Geometry check sheet. Reference: drawing and pictorial views, mm from the part's lowest x, y, z. Give positions to 0.01 mm unless a question says otherwise; leave off trailing zeros. Write each loop counter-clockwise with the first axis right and the second up, starting at its lowest first coordinate (ties: lowest second). Pieces come first, ordered by that corner, then holes. Notation, with made-up numbers: (-9.75, -20) -> (1.25, -20) arc R13 cw to (1.25, 0) -> close; hole circle Ø5 at (37.25, -23.5). An arc over 180 degrees is marked (long way). Write each question's results on one line, items separated by ' | '. Start each with the question number.
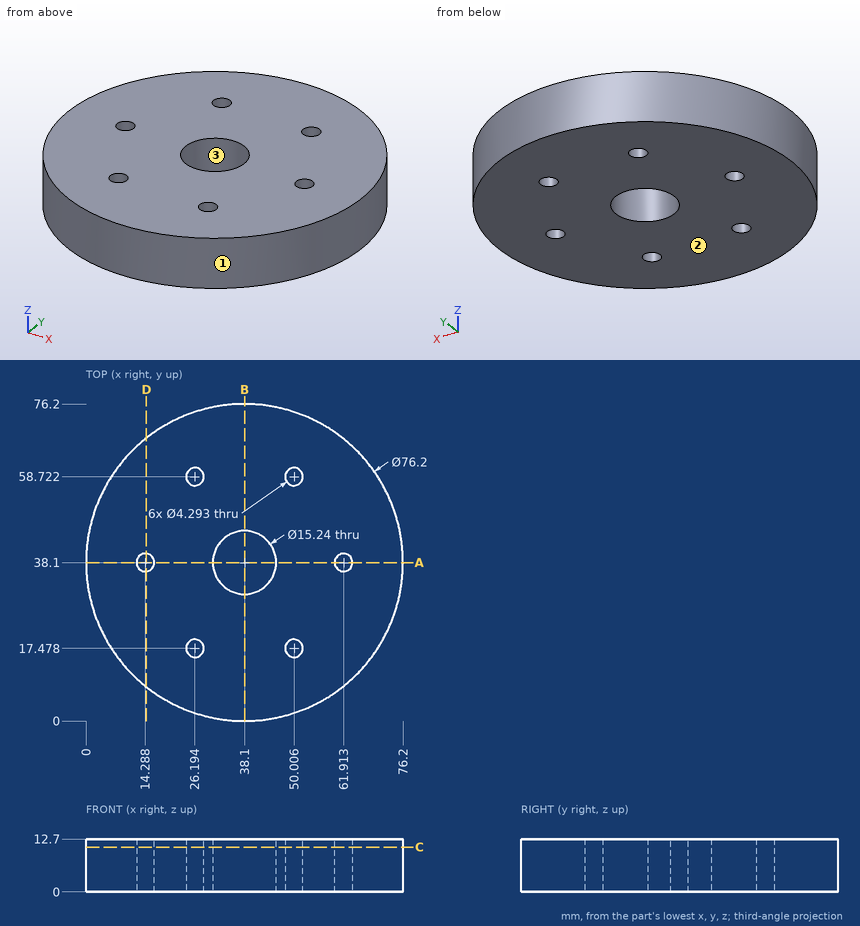
Item 1: Section check B-B on x = 38.1. Record the boundary of the cut face in (y, z).
Item 2: Section check D-D on x = 14.5. Record the boundary of the cut face in (y, z) (1 decimal).
Item 3: Depth check by flat-ended pin: pin 1 Ø4 at (x, z) = (27, 2) entering from -Y; pin 2 Ø3.5 at (x, y) = (50.01, 58.72) entering from -Z; pin 3 Ø5 at (x, y) = (50.01, 17.48) entering from -Z; pin 4 Ø1 at (y, z) = (52, 1.5) entering from -X (1 decimal). Enter the tip coordinate at first touch or a pass-through.
Item 4: Mould release check, pull along X, two halves, no side actions. Record for the marked faces 1, 2 and 3: pulls with the +X half, pulls with the -X half, needs draft (parallel to the pull), parting line crosses it, or undercut.
Item 5: Section check C-C on z = 10.75. Record the boundary of the cut face in (x, y).
Item 6: Section check A-A on y = 38.1. Record the boundary of the cut face in (x, z).
Item 7: Thickness scan on probe 1 along Y at (x, z) = (38, 4.5); probe 2 along X at (y, z) = (19, 11.75) (1 decimal); probe 3 along Y at (x, z) = (27, 8.5). Record the ranges inside material, lowest first. Write a range as from..to.
Check sheet entries:
1) outline: (0, 0) -> (30.48, 0) -> (30.48, 12.7) -> (0, 12.7) -> close; (45.72, 0) -> (76.2, 0) -> (76.2, 12.7) -> (45.72, 12.7) -> close
2) outline: (8.2, 0) -> (36, 0) -> (36, 12.7) -> (8.2, 12.7) -> close; (40.2, 0) -> (68, 0) -> (68, 12.7) -> (40.2, 12.7) -> close
3) pin 1: stops at y = 1.1 | pin 2: passes through | pin 3: stops at z = 0 | pin 4: stops at x = 2.4
4) face 1: parting line crosses it | face 2: needs draft | face 3: undercut
5) outline: circle Ø76.2 at (38.1, 38.1); hole circle Ø4.29 at (14.29, 38.1); hole circle Ø4.29 at (26.19, 17.48); hole circle Ø4.29 at (26.19, 58.72); hole circle Ø15.24 at (38.1, 38.1); hole circle Ø4.29 at (50.01, 17.48); hole circle Ø4.29 at (50.01, 58.72); hole circle Ø4.29 at (61.91, 38.1)
6) outline: (0, 0) -> (12.14, 0) -> (12.14, 12.7) -> (0, 12.7) -> close; (16.43, 0) -> (30.48, 0) -> (30.48, 12.7) -> (16.43, 12.7) -> close; (45.72, 0) -> (59.77, 0) -> (59.77, 12.7) -> (45.72, 12.7) -> close; (64.06, 0) -> (76.2, 0) -> (76.2, 12.7) -> (64.06, 12.7) -> close
7) probe 1: y = 0..30.48, 45.72..76.2 | probe 2: x = 5.1..24.7, 27.7..48.5, 51.5..71.1 | probe 3: y = 1.65..15.49, 19.47..56.73, 60.71..74.55
